The listing builds one solid part. Answer for the finished solid, in the listing's coordinates (mm). Round coordinates to 2 decimals unless told otherwise and drop trailing zeros. Write each loop counter-clockwise with the first axis right and the second up, starting at its lowest first coordinate (ties: lowest second). Pieces come first, ordered by that corner, then holes.
from build123d import *

# Parameters (mm, degrees)
F0_W     = 12.115448
F0_H     = 9.97743
F0_W_2   = 56.370701
F0_H_2   = 3.390066
F0_R     = 2.542431
F0_W_3   = 18.290117
F0_H_3   = 5
F1_DEPTH = 5


with BuildPart() as f1:
    # F0 (on Top) → F1 (new body)
    with BuildSketch(Plane.XY):
        Polygon((-115.620404, 83.065476), (-121.425346, 83.065476), (-121.425346, -88.866214), (-115.620404, -88.866214), (-97.330287, -88.866214), (8.093566, -88.866214), (26.383683, -88.866214), (32.188624, -88.866214), (32.188624, 83.065476), (26.383683, 83.065476), (8.093566, 83.065476), (-91.525346, 83.065476), (-97.330287, 83.065476), align=None)
        with Locations((-104.766935, -71.978614)):
            Rectangle(F0_W, F0_H, mode=Mode.SUBTRACT)
        with Locations((-104.766935, -56.598406)):
            Rectangle(F0_W, F0_H, mode=Mode.SUBTRACT)
        with Locations((-104.766935, -42.02375)):
            Rectangle(F0_W, F0_H, mode=Mode.SUBTRACT)
        with Locations((15.530214, -71.978614)):
            Rectangle(F0_W, F0_H, mode=Mode.SUBTRACT)
        with Locations((15.530214, -56.598406)):
            Rectangle(F0_W, F0_H, mode=Mode.SUBTRACT)
        with Locations((-44.61836, -29.415544)):
            Rectangle(F0_W_2, F0_H_2, mode=Mode.SUBTRACT)
        with Locations((15.530214, -42.02375)):
            Rectangle(F0_W, F0_H, mode=Mode.SUBTRACT)
        with Locations((-104.766935, 36.223011)):
            Rectangle(F0_W, F0_H, mode=Mode.SUBTRACT)
        with Locations((-104.766935, 50.797667)):
            Rectangle(F0_W, F0_H, mode=Mode.SUBTRACT)
        with Locations((-104.766935, 66.177875)):
            Rectangle(F0_W, F0_H, mode=Mode.SUBTRACT)
        with Locations((-44.618361, -2.900369)):
            Circle(F0_R, mode=Mode.SUBTRACT)
        with Locations((-44.61836, 23.614805)):
            Rectangle(F0_W_2, F0_H_2, mode=Mode.SUBTRACT)
        with Locations((15.530214, 36.223011)):
            Rectangle(F0_W, F0_H, mode=Mode.SUBTRACT)
        with Locations((15.530214, 50.797667)):
            Rectangle(F0_W, F0_H, mode=Mode.SUBTRACT)
        with Locations((15.530214, 66.177875)):
            Rectangle(F0_W, F0_H, mode=Mode.SUBTRACT)
        with Locations((-106.475346, 85.565476)):
            Rectangle(F0_W_3, F0_H_3)
        with Locations((-106.475346, -91.366214)):
            Rectangle(F0_W_3, F0_H_3)
        with Locations((17.238625, -91.366214)):
            Rectangle(F0_W_3, F0_H_3)
        with Locations((17.238625, 85.565476)):
            Rectangle(F0_W_3, F0_H_3)
    extrude(amount=F1_DEPTH)


solid = f1.part
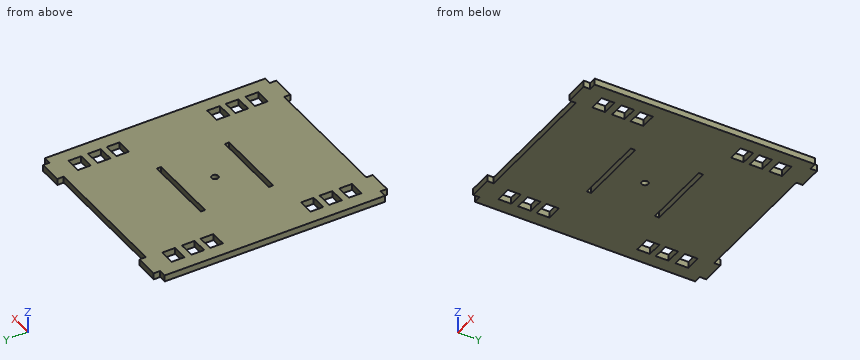
1. Section B-B on y = 69 is taken. Determine the outline of the cut face in (x, z), plus the area to 3 significant figures.
Geometry says:
outline: (-121.43, 0) - (-110.82, 0) - (-110.82, 5) - (-121.43, 5) - close; (-98.71, 0) - (9.47, 0) - (9.47, 5) - (-98.71, 5) - close; (21.59, 0) - (32.19, 0) - (32.19, 5) - (21.59, 5) - close
area: 647 mm2
2. Section A-A on x = 16.5 is taken. Determine the outline of the cut face in (y, z).
Geometry says:
outline: (-93.87, 0) - (-76.97, 0) - (-76.97, 5) - (-93.87, 5) - close; (-66.99, 0) - (-61.59, 0) - (-61.59, 5) - (-66.99, 5) - close; (-51.61, 0) - (-47.01, 0) - (-47.01, 5) - (-51.61, 5) - close; (-37.04, 0) - (31.23, 0) - (31.23, 5) - (-37.04, 5) - close; (41.21, 0) - (45.81, 0) - (45.81, 5) - (41.21, 5) - close; (55.79, 0) - (61.19, 0) - (61.19, 5) - (55.79, 5) - close; (71.17, 0) - (88.07, 0) - (88.07, 5) - (71.17, 5) - close
3. Given pin 1 (1 mm diameter, centred on x = -62, z = 2, fed in from +Y); pin 2 (1 mm diameter, centred on x = -29.5, z = 3, fed in from -Y); pin 3 (1.5 mm diameter, centred on y = 85.5, z = 3, fed in from +X), each flat-ended and moving along its own axis, determine where each tip first touches the part or whether it passes through.
Geometry says:
pin 1: stops at y = 83.07
pin 2: stops at y = -88.87
pin 3: stops at x = 26.38
4. Section D-D on z = 1.45 is taken. Give the number of separate pieces and of enclosed holes in the cut face, plus the area to 3 significant figures.
Geometry says:
separate pieces: 1
enclosed holes: 15
area: 24,900 mm2
5. Straight lines are drawn through the part: line 1 along X through (y, z) = (53.5, 1.7); line 2 along Y through (x, z) = (-19.5, 3.7); line 3 along Y through (x, z) = (-8.5, 1.75). For each, find the intervals that lie inside material, in ascending order.
Geometry says:
line 1: x = -121.43 to -110.82, -98.71 to 9.47, 21.59 to 32.19
line 2: y = -88.87 to -31.11, -27.72 to 21.92, 25.31 to 83.07
line 3: y = -88.87 to 83.07
6. Section C-C on x = -53.5 is taken. Determine the outline of the cut face in (y, z), plus the area to 3 significant figures.
Geometry says:
outline: (-88.87, 0) - (-31.11, 0) - (-31.11, 5) - (-88.87, 5) - close; (-27.72, 0) - (21.92, 0) - (21.92, 5) - (-27.72, 5) - close; (25.31, 0) - (83.07, 0) - (83.07, 5) - (25.31, 5) - close
area: 826 mm2
